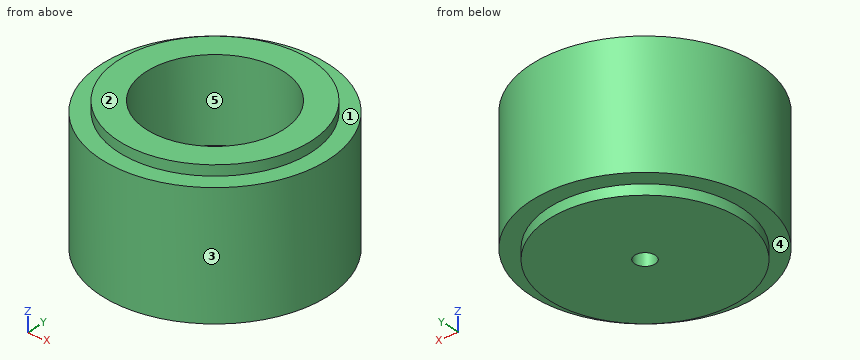
```python
from build123d import *

# Parameters (mm, degrees)
SKETCH1_R           = 14
SKETCH1_R_2         = 1.5
BOSS_EXTRUDE1_DEPTH = 1.5
SKETCH2_R           = 10.5
SKETCH2_R_2         = 1.5
BOSS_EXTRUDE2_DEPTH = 18
SKETCH3_R           = 14
SKETCH3_R_2         = 1.5
BOSS_EXTRUDE3_DEPTH = 1.5
SKETCH4_R           = 10
CUT_EXTRUDE1_DEPTH  = 12
SKETCH5_R           = 16.5
SKETCH5_R_2         = 10.5
BOSS_EXTRUDE4_DEPTH = 18


with BuildPart() as part:
    # Sketch1 → Boss-Extrude1 (new body)
    with BuildSketch(Plane.XY):
        Circle(SKETCH1_R)
        Circle(SKETCH1_R_2, mode=Mode.SUBTRACT)
    extrude(amount=BOSS_EXTRUDE1_DEPTH)

    # Sketch2 → Boss-Extrude2 (add)
    with BuildSketch(Plane.XY.offset(1.5)):
        Circle(SKETCH2_R)
        Circle(SKETCH2_R_2, mode=Mode.SUBTRACT)
    extrude(amount=BOSS_EXTRUDE2_DEPTH)

    # Sketch3 → Boss-Extrude3 (add)
    with BuildSketch(Plane.XY.offset(19.5)):
        Circle(SKETCH3_R)
        Circle(SKETCH3_R_2, mode=Mode.SUBTRACT)
    extrude(amount=BOSS_EXTRUDE3_DEPTH)

    # Sketch4 → Cut-Extrude1 (cut)
    with BuildSketch(Plane.XY.offset(21)):
        Circle(SKETCH4_R)
    extrude(amount=-CUT_EXTRUDE1_DEPTH, mode=Mode.SUBTRACT)

    # Sketch5 → Boss-Extrude4 (add)
    with BuildSketch(Plane.XY.offset(1.5)):
        Circle(SKETCH5_R)
        Circle(SKETCH5_R_2, mode=Mode.SUBTRACT)
    extrude(amount=BOSS_EXTRUDE4_DEPTH)


solid = part.part
```
Input: part model. Units: mm. Frame: model coordinates. Face numbers are marked on the shaded views. A direction names the side the tool comes from. Give positions to 0.01 mm unless a question says otherwise; leave off trailing zeros. Order: outer loops, then holes, each group sorted by start corner. A loop starts at its lowest first (then second) coordinate and runs counter-clockwise, first axis right, second up. Notation, with made-up numbers: M 53.5,59.5 L 104.5,59.5 A28 cw 104.5,86.5 Z; hole C -39,21.25 d2. An arc over 180 degrees is marked long. Return JSON: item names as keys, results as strings.
Item 1: Access query for the marked faces 1 and 2. Directions: +Z, -Z, +X, -X, +Y, -Y. A direction counts if a zero-diameter tool reaches every point of the face in a straight line with its end or side. Return the directions, or none.
Solutions:
{"face 1": "+Z", "face 2": "+Z, +X, -X, +Y, -Y"}
Item 2: Cut plane A-A (x = 0). Return loops of the section in (y, z).
Solutions:
{"outline": "M -16.5,1.5 L -14,1.5 L -14,0 L -1.5,0 L -1.5,9 L -10,9 L -10,21 L -14,21 L -14,19.5 L -16.5,19.5 Z; M 1.5,0 L 14,0 L 14,1.5 L 16.5,1.5 L 16.5,19.5 L 14,19.5 L 14,21 L 10,21 L 10,9 L 1.5,9 Z"}
Item 3: Cut plane D-D (y = -12). Return loops of the section in (x, z).
Solutions:
{"outline": "M -11.32,1.5 L -7.21,1.5 L -7.21,0 L 7.21,0 L 7.21,1.5 L 11.32,1.5 L 11.32,19.5 L 7.21,19.5 L 7.21,21 L -7.21,21 L -7.21,19.5 L -11.32,19.5 Z"}
Item 4: Ray query, probe 1 along Y at (x, z) = (0, 4.75); probe 2 along Y at (x, z) = (0, 17.75); probe 3 along X at (y, z) = (-8, 19). Return the intervals inside material, ascending.
Solutions:
{"probe 1": "-16.5 to -1.5, 1.5 to 16.5", "probe 2": "-16.5 to -10, 10 to 16.5", "probe 3": "-14.43 to -6, 6 to 14.43"}
Item 5: Cut plane C-C (z = 11.5). Return loops of the section in (x, y), then the cut area to 3 significant figures.
Solutions:
{"outline": "C 0,0 d33; hole C 0,0 d20", "area": "541 mm^2"}
Item 6: Pull-direction query (X, two-part tool) for the marked faces 3, 4 and 5; classes: +X half, -X half, draft (parallel to the pull), parting line (faces both ways), or undercut.
Solutions:
{"face 3": "parting line", "face 4": "draft", "face 5": "undercut"}
Item 7: First-contact query: P1, Ø6, axis at x = 5, z = 2.5, coming from the -Y side; P2, Ø12, axis at x = -7, y = -10, coming from the -Z side; P3, Ø1.5, axis at y = -12.5, z = 11.5, coming from the +X side; P4, Ø6, axis at y = -13, z = 7.5, coming from the +X side. Flat tips, straight axial feed; report the tip coordinate or a pass-through.
Solutions:
{"P1": "y = -16.38", "P2": "z = 0", "P3": "x = 11.58", "P4": "x = 13.12"}
